from build123d import *

# Parameters (mm, degrees)
FILLET1_R          = 0.25
CUT_EXTRUDE1_DEPTH = 15.2


with BuildPart() as part:
    # Sketch2 → Revolve1 (revolve)
    with BuildSketch(Plane(origin=(0, 0, 0), x_dir=(0, 0, -1), z_dir=(1, 0, 0))):
        Polygon((0, 0), (2.5, 0), (2.5, 5.2), (1.4, 5.2), (1.4, 20.4), (0, 20.4), align=None)
    revolve(axis=Axis((0, 20.4, 0), (0, -1, 0)))

    # Fillet1
    fillet1_edges = [part.edges().sort_by_distance(p)[0] for p in [
        (0, 0, 2.5),
    ]]
    fillet(fillet1_edges, radius=FILLET1_R)

    # Sketch3 → Cut-Extrude1 (cut)
    with BuildSketch(Plane(origin=(0, 20.4, 0), x_dir=(1, 0, 0), z_dir=(0, 1, 0))):
        with BuildLine():
            Line((1.09287465, -0.875), (-1.09287465, -0.875))
            ThreePointArc((-1.09287465, -0.875), (0, -1.4), (1.09287465, -0.875))
        make_face()
    extrude(amount=-CUT_EXTRUDE1_DEPTH, mode=Mode.SUBTRACT)


solid = part.part
Model file for the job. Use its own axes, mm. A direction names the side the tool comes from. Coordinates: 2 decimals unless noted, no trailing zeros. Order: outer loops, then holes, each group sorted by start corner. A loop starts at its lowest first (then second) coordinate and runs counter-clockwise, first axis right, second up. Notation, with made-up numbers: (13.5, 28) -> (23.5, 28) arc R26 cw to (23.5, 45) -> close; hole circle Ø5 at (75, 23). An arc over 180 degrees is marked (long way). Return JSON: item names as keys, results as strings. Group by question number.
Item 1: Saw through at D-D on y = 5.75. Write the cut outline in (x, z) (3 decimals), then the cut area to 3 significant figures.
Item 2: Flat gauge pins, fed straight in: P1, Ø0.7, axis at x = 0.5, y = 12.5, coming from the +Z side (3 decimals); P2, Ø1.5, axis at y = 14.5, z = 2, coming from the +X side. Where does each tip first touch, or does it go through?
Item 3: Tool access for faces 1 (the flat face through (0, 5.2, 1.1)), 2 (the flat face through (0, 13, 0.875)), 3 (the cylindrical face through (-2.44, 2.76, 0.54)): list every direction of +Z, -Z, +X, -X, +Y, -Y with a clear straight run to the whole face (end or side of a thin tool).
Item 4: Saw through at C-C on y = 3.5. Write the cut outline in (x, z).
Item 5: Saw through at A-A on z = 0. Write the cut outline in (x, y), then the cut area to 3 significant figures.
Item 6: Saw through at B-B on x = 0. Write the cut outline in (y, z) (3 decimals), then the cut area to 3 significant figures.
Item 7: Wall check: line 1 along Y through (x, z) = (-1.8, -0.35); line 2 along Z through (x, y) = (-0.1, 9.5) (3 decimals); line 3 along X through (y, z) = (11.25, 0.35). Give the ranges that are in metal, low to high. Write a range as [from, to].
Values found:
{
 "1": {"outline": "(-1.093, 0.875) arc R1.4 ccw (long way) to (1.093, 0.875) -> close", "area": "5.36 mm2"},
 "2": {"P1": "stops at z = 0.875", "P2": "passes through"},
 "3": {"face 1": "+Y", "face 2": "+Z, +X, -X, +Y", "face 3": "+Y, -Y"},
 "4": {"outline": "circle Ø5 at (0, 0)"},
 "5": {"outline": "(-2.5, 0.25) arc R0.25 ccw to (-2.25, 0) -> (2.25, 0) arc R0.25 ccw to (2.5, 0.25) -> (2.5, 5.2) -> (1.4, 5.2) -> (1.4, 20.4) -> (-1.4, 20.4) -> (-1.4, 5.2) -> (-2.5, 5.2) -> close", "area": "68.5 mm2"},
 "6": {"outline": "(0, -2.25) arc R0.25 ccw to (0.25, -2.5) -> (5.2, -2.5) -> (5.2, -1.4) -> (20.4, -1.4) -> (20.4, 0.875) -> (5.2, 0.875) -> (5.2, 2.5) -> (0.25, 2.5) arc R0.25 ccw to (0, 2.25) -> close", "area": "60.6 mm2"},
 "7": {"line 1": "y = [0, 5.2]", "line 2": "z = [-1.396, 0.875]", "line 3": "x = [-1.36, 1.36]"}
}
